from build123d import *

# Parameters (mm, degrees)
SKETCH1_W             = 193.548
SKETCH1_H             = 172.974
BASE_DEPTH            = 4.826
CENTER_CUT_DEPTH      = 260.623040688
LEADING_EDGE_FILLET_R = 12.7


with BuildPart() as part:
    # Sketch1 → Base (new body)
    with BuildSketch(Plane(origin=(0, 0, 0), x_dir=(1, 0, 0), z_dir=(0, 1, 0))):
        with Locations((96.774, 86.487)):
            Rectangle(SKETCH1_W, SKETCH1_H)
    extrude(amount=BASE_DEPTH)

    # Sketch2 → Center Cut (cut, through all)
    with BuildSketch(Plane(origin=(0, 4.826, 0), x_dir=(1, 0, 0), z_dir=(0, 1, 0))):
        with BuildLine():
            Line((20.574, 101.6), (14.224, 172.974))
            Line((14.224, 172.974), (179.324, 172.974))
            Line((179.324, 172.974), (172.974, 101.6))
            ThreePointArc((172.974, 101.6), (96.774, 25.4), (20.574, 101.6))
        make_face()
    extrude(amount=-CENTER_CUT_DEPTH, mode=Mode.SUBTRACT)

    # Leading Edge Fillet
    leading_edge_fillet_edges = [part.edges().sort_by_distance(p)[0] for p in [
        (14.224, 2.413, -172.974),
        (179.324, 2.413, -172.974),
    ]]
    fillet(leading_edge_fillet_edges, radius=LEADING_EDGE_FILLET_R)


solid = part.part
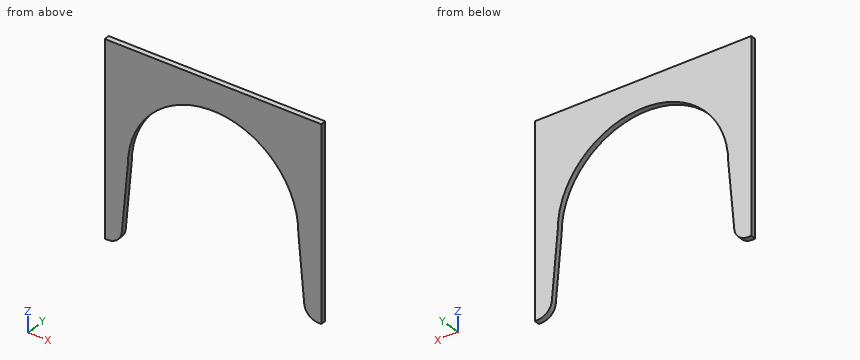
Model file for the job. Use its own axes, mm. Round coordinates to 2 decimals unless told otherwise and drop trailing zeros. Loops run counter-clockwise (first coordinate to the right, second up) from the corner with the lowest first, then second, coordinate; pieces in that order, holes last.
1. Band-saw the part on D-D, the plane x = 162.5. List the corners of the cut face in (y, z).
Check values:
outline: (0, -63.04) - (4.83, -63.04) - (4.83, 0) - (0, 0) - close
2. Drop flat-ended pins along their axis: P1, Ø1, axis at x = 91.5, y = 4, coming from the -Z side; P2, Ø2, axis at x = 107.5, y = 1, coming from the -Z side. Give the stop position or say it passes through.
Check values:
P1: stops at z = -25.62
P2: stops at z = -26.31
3. Band-saw the part on A-A, the plane z = -84. List the corners of the cut face in (x, y).
Check values:
outline: (0, 0) - (22.63, 0) - (22.63, 4.83) - (0, 4.83) - close; (170.91, 0) - (193.55, 0) - (193.55, 4.83) - (170.91, 4.83) - close
4. Wall check: probe 1 along X at (y, z) = (4.3, -33); probe 2 along X at (y, z) = (3.55, -135); probe 3 along Z at (x, y) = (79.5, 4.5). Give the ranges that are in metal, low to high.
Check values:
probe 1: x = 0 to 63.6, 129.95 to 193.55
probe 2: x = 0 to 17.6, 175.95 to 193.55
probe 3: z = -27.38 to 0
5. Band-saw the part on C-C, the plane z = -36. List the corners of the cut face in (x, y).
Check values:
outline: (0, 0) - (58, 0) - (58, 4.83) - (0, 4.83) - close; (135.54, 0) - (193.55, 0) - (193.55, 4.83) - (135.54, 4.83) - close
6. Band-saw the part on B-B, the plane y = 2.15. List the corners of the cut face in (x, z), and give its area (3 significant figures).
Check values:
outline: (0, -172.97) - (2.6, -172.97) arc R12.7 ccw to (15.25, -161.4) - (20.57, -101.6) arc R76.2 cw to (172.97, -101.6) - (178.29, -161.4) arc R12.7 ccw to (190.94, -172.97) - (193.55, -172.97) - (193.55, 0) - (0, 0) - close
area: 13,000 mm2
